Part print with two shaded views. Sizes in mm from the minimum x, y, z corner. Round coordinates to 2 decimals unless told otherwise and drop trailing zeros. Order: outer loops, then holes, each group sorted by start corner. A loop starts at its lowest first (then second) coordinate and runs counter-clockwise, first axis right, second up. Notation, with made-up numbers: M 25,9 L 36,9 A25 cw 36,37 Z; hole C 18,72.25 d5. An arc over 180 degrees is marked long. Answer as a JSON object with one key per item and string values.
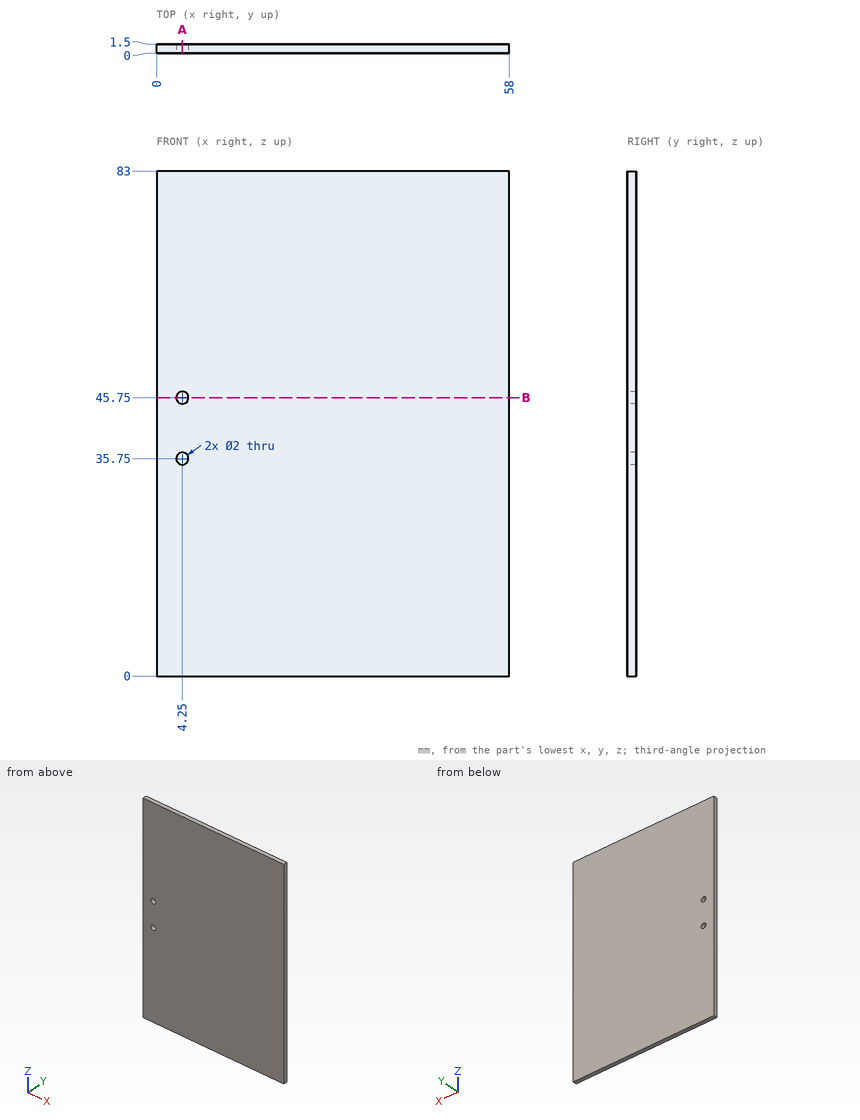
Item 1: Saw through at B-B on z = 45.75. List the corners of the cut face in (x, y), and give its area (3 significant figures).
Worked answers:
{"outline": "M 0,0 L 3.25,0 L 3.25,1.5 L 0,1.5 Z; M 5.25,0 L 58,0 L 58,1.5 L 5.25,1.5 Z", "area": "84.0 mm2"}
Item 2: Wall check: line 1 along Z through (x, y) = (4.25, 0.9); line 2 along X through (y, z) = (0.6, 45.75). Give the ranges that are in metal, low to high. Write a range as [from, to].
Worked answers:
{"line 1": "z = [0, 34.75], [36.75, 44.75], [46.75, 83]", "line 2": "x = [0, 3.25], [5.25, 58]"}
Item 3: Saw through at A-A on x = 4.25. List the corners of the cut face in (y, z), and give its area (4 significant figures).
Worked answers:
{"outline": "M 0,0 L 1.5,0 L 1.5,34.75 L 0,34.75 Z; M 0,36.75 L 1.5,36.75 L 1.5,44.75 L 0,44.75 Z; M 0,46.75 L 1.5,46.75 L 1.5,83 L 0,83 Z", "area": "118.5 mm2"}
